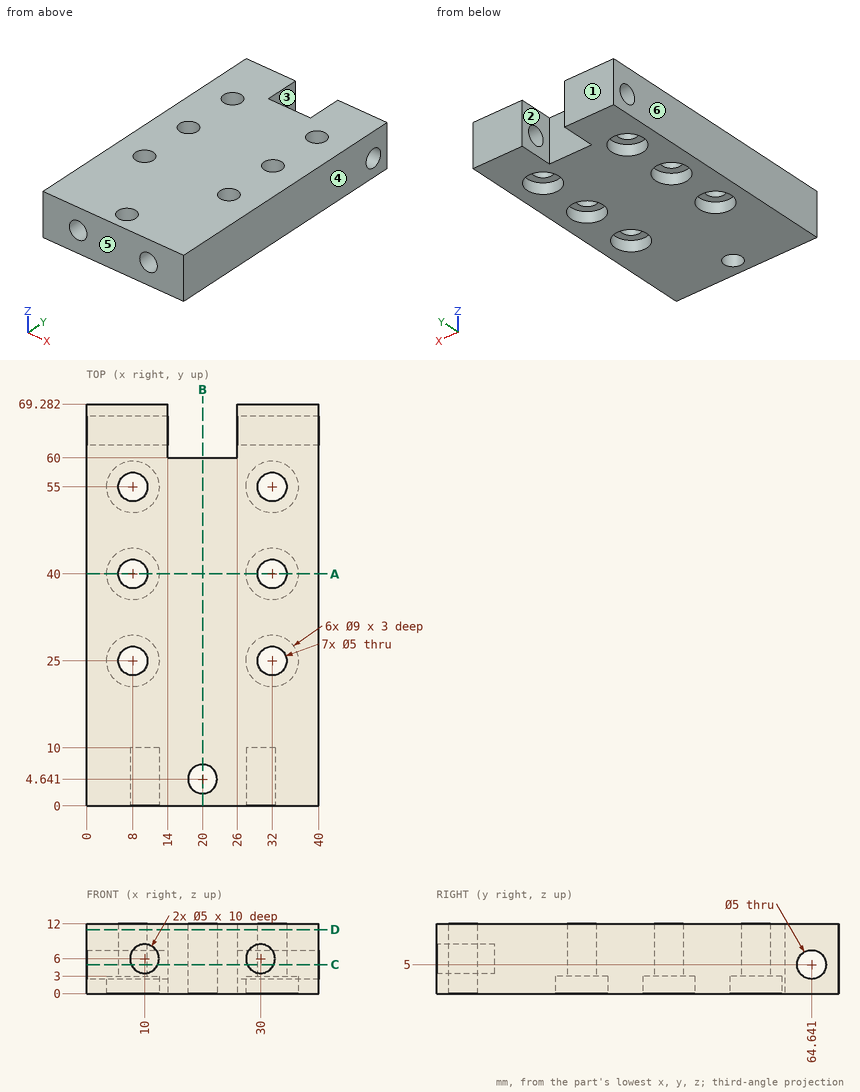
Check sheet for the drawn part. Datum: minimum x, y, z corner. Units: mm. A direction names the side the tool comes from. Round coordinates to 2 decimals unless told otherwise and drop trailing zeros. Loops run counter-clockwise (first coordinate to the right, second up) from the corner with the lowest first, then second, coordinate; pieces in that order, holes last. Notation, with made-up numbers: (-5.75, -6.75) - (48.25, -6.75) arc R25 cw to (48.25, 10.25) - close; hole circle Ø9 at (-1, 75). An arc over 180 degrees is marked (long way). Write item = value, one per line. Start each with the question number.
1. Depth check by flat-ended pin: pin 1 (1.5 mm diameter, centred on x = 10.5, z = 6.5, fed in from -Y); pin 2 (5 mm diameter, centred on x = 17, z = 5.5, fed in from +Y). Enter the tip coordinate at first touch or a pass-through.
2. Thickness scan on line 1 (Y direction, x = 8, z = 5); line 2 (Y direction, x = 8, z = 9.25); line 3 (Y direction, x = 32, z = 1.35). Record the ranges inside material, lowest first.
3. Section check D-D on z = 11. Enter the section's corners in (x, y), then the cut area to 3 significant figures.
4. Section check C-C on z = 5. Give the number of separate pieces and of enclosed holes in the cut face, then the cut area to 3 significant figures.
5. Section check B-B on x = 20. Enter the section's corners in (y, z).
6. Set-up check for the marked faces 1 and 2: record each of +Z, -Z, +X, -X, +Y, -Y from which the full face is reachable in a straight line by a thin tool's end or side.
7. Mould release check, pull along X, two halves, no side actions. Record for the marked faces 3, 4, 5 and 6: released by +X, released by -X, zero draft, split by the parting line, or undercut.
8. Section check A-A on y = 40. Enter the section's corners in (x, z).
Working result:
q1.pin_1 = 10
q1.pin_2 = 60
q2.line_1 = 10 to 22.5, 27.5 to 37.5, 42.5 to 52.5, 57.5 to 62.14, 67.14 to 69.28
q2.line_2 = 0 to 22.5, 27.5 to 37.5, 42.5 to 52.5, 57.5 to 69.28
q2.line_3 = 0 to 20.5, 29.5 to 35.5, 44.5 to 50.5, 59.5 to 69.28
q3.outline = (0, 0) - (40, 0) - (40, 69.28) - (26, 69.28) - (26, 60) - (14, 60) - (14, 69.28) - (0, 69.28) - close; hole circle Ø5 at (8, 25); hole circle Ø5 at (8, 40); hole circle Ø5 at (8, 55); hole circle Ø5 at (20, 4.64); hole circle Ø5 at (32, 25); hole circle Ø5 at (32, 40); hole circle Ø5 at (32, 55)
q3.area = 2,520 mm^2
q4.separate_pieces = 3
q4.enclosed_holes = 7
q4.area = 2,290 mm^2
q5.outline = (0, 0) - (2.14, 0) - (2.14, 12) - (0, 12) - close; (7.14, 0) - (60, 0) - (60, 12) - (7.14, 12) - close
q6.face_1 = +Z, -Z, +X, -X, +Y
q6.face_2 = +Z, -Z, +Y
q7.face_3 = undercut
q7.face_4 = released by +X
q7.face_5 = zero draft
q7.face_6 = released by -X
q8.outline = (0, 0) - (3.5, 0) - (3.5, 3) - (5.5, 3) - (5.5, 12) - (0, 12) - close; (10.5, 3) - (12.5, 3) - (12.5, 0) - (27.5, 0) - (27.5, 3) - (29.5, 3) - (29.5, 12) - (10.5, 12) - close; (34.5, 3) - (36.5, 3) - (36.5, 0) - (40, 0) - (40, 12) - (34.5, 12) - close
